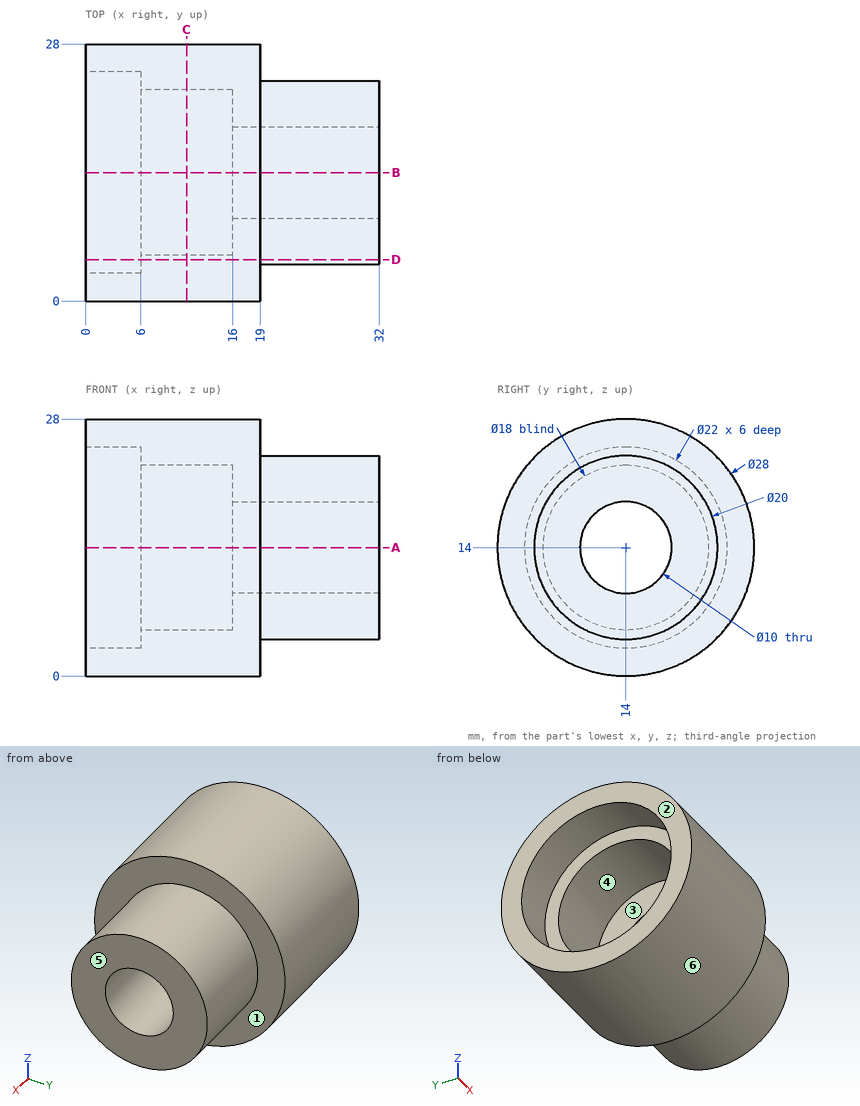
The drawing under review shows one solid part. Ordinate dimensions are in mm from its lowest x, y, z. A direction names the side the tool comes from. Coordinates: 2 decimals unless noted, no trailing zeros. Write each loop counter-clockwise with the first axis right and the second up, starting at its lowest first coordinate (ties: lowest second). Pieces come first, ordered by that corner, then holes. Notation, with made-up numbers: (11.25, 62.25) -> (26.25, 62.25) arc R30 ccw to (26.25, 97.25) -> close; hole circle Ø7 at (54.25, -4.75). An arc over 180 degrees is marked (long way). Write each question's results on one line, items separated by ' | '. Start each with the question number.
1) For the marked faces 1, 2 and 3, list the 3-axis set-ups (+Z, -Z, +X, -X, +Y, -Y) from which the entire face can be reached by the end or side of a thin tool; tool diameter is ignored.
2) Wall thickness on L1, parallel to Y at x = 21.75, z = 14; L2, parallel to X at y = 18, z = 19.5; L3, parallel to Y at x = 2.5, z = 14.25: over which ranges is each line inside the solid? List them lowest first. Write a range as [from, to].
3) The part is to be moulded in two halves that separate along Z. For the marked faces 4, 5 and 6, say which applies: +Z half, -Z half, draft (parallel to the pull), parting line (faces both ways), or undercut.
4) Consider section C-C (x = 11). Write out the cut boundary in (y, z), plus the area to 3 significant figures.
5) Consider section D-D (y = 4.5). Write out the cut boundary in (x, z).
6) Insertion check: pin 1 (1 mm diameter, centred on y = 24.5, z = 18.5, fed in from -X); pin 2 (4 mm diameter, centred on x = 10, y = 8.5, fed in from -Z); pin 3 (9 mm diameter, centred on y = 15, z = 11.5, fed in from -X); pin 4 (9 mm diameter, centred on y = 14, z = 14, fed in from +X). Each pin has a flat end and moves straight along its axis. Give the tip position at first contact, or say it passes through.
7) Consider section A-A (z = 14). Write out the cut boundary in (x, y), plus the area to 3 significant figures.
Geometry says:
1) face 1: +X | face 2: +Z, -Z, -X, +Y, -Y | face 3: -X
2) L1: [4, 9], [19, 24] | L2: [16, 32] | L3: [0, 3], [25, 28]
3) face 4: undercut | face 5: draft | face 6: parting line
4) outline: circle Ø28 at (14, 14); hole circle Ø18 at (14, 14) | area: 361 mm^2
5) outline: (0, 3.72) -> (19, 3.72) -> (19, 10.88) -> (32, 10.88) -> (32, 17.12) -> (19, 17.12) -> (19, 24.28) -> (0, 24.28) -> (0, 19.55) -> (6, 19.55) -> (6, 8.45) -> (0, 8.45) -> close
6) pin 1: x = 0 | pin 2: z = 0.44 | pin 3: x = 16 | pin 4: through
7) outline: (0, 0) -> (19, 0) -> (19, 4) -> (32, 4) -> (32, 9) -> (16, 9) -> (16, 5) -> (6, 5) -> (6, 3) -> (0, 3) -> close; (0, 25) -> (6, 25) -> (6, 23) -> (16, 23) -> (16, 19) -> (32, 19) -> (32, 24) -> (19, 24) -> (19, 28) -> (0, 28) -> close | area: 320 mm^2
